Design review of the part built by this model. Coordinates are the model's own, in mm. A direction names the side the tool comes from. Coordinates: 2 decimals unless noted, no trailing zeros. Loops run counter-clockwise (first coordinate to the right, second up) from the corner with the lowest first, then second, coordinate; pieces in that order, holes last. Notation, with made-up numbers: M 40,31.25 L 76,31.25 A12 cw 76,53.25 Z; hole C 7,21 d2. An arc over 180 degrees is marked long. Put each result on its own line as item: value. Start each with the question number.
(1) Take a section at C-C, the plane z = -5.75. Give the boundary of the cut face in (x, y) (3 decimals), then the cut area to 3 significant figures.
(2) Clearance check with flat-ended pins moving along their axes: pin 1 (6 mm diameter, centred on x = -1, y = 2, fed in from +Z); pin 2 (1.5 mm diameter, centred on x = -0.5, z = 14, fed in from -Y); pin 3 (0.9 mm diameter, centred on y = 10, z = -11.5, fed in from -X); pin 4 (1.5 mm diameter, centred on y = 10.5, z = -11.5, fed in from +X). State where each tip first meets the part, or that it passes through.
(3) For probe 1 along Z at (x, y) = (-3, 7.25); probe 2 along Y at (x, z) = (1.5, -5); probe 3 along X at (y, z) = (2.2, 8), list the stretches that pass through material, from the lowest coordinate up. Write a range as [from, to].
(4) Take a section at D-D, the plane y = 10.75. Give the boundary of the cut face in (x, z).
(5) Take a section at A-A, the plane x = -5.5. Give the boundary of the cut face in (y, z), then the cut area to 3 significant figures.
(6) The part is to be moulded in two halves that separate along Z. For faces 1 (the cylindrical face through (1.142, -1.792, -0.182)), 2 (the flat face through (-2, 3.315, 7)), 3 (the flat face through (2, 2, 13)), say which applies: +Z half, -Z half, draft (parallel to the pull), parting line (faces both ways), or undercut.
(7) For faces 4 (the flat face through (-2, 11, -12)), 5 (the flat face through (0, 3.75, 14)), 6 (the cylindrical face through (-1.08, -4.88, -4.93)), list the 3-axis set-ups (+Z, -Z, +X, -X, +Y, -Y) from which the entire face can be reached by the end or side of a thin tool; tool diameter is ignored.
(8) Take a section at B-B, the plane y = -0.75. Give the boundary of the cut face in (x, z), then the cut area to 3 significant figures.
Autodesk Inventor part; units mm, degrees
ref_plane "YZ Plane" through (0, 0, 0) normal (1, 0, 0) x (0, 1, 0)
ref_plane "XZ Plane" through (0, 0, 0) normal (0, 1, 0) x (-1, 0, 0)
ref_plane "XY Plane" through (0, 0, 0) normal (0, 0, 1) x (1, 0, 0)
sketch "Sketch1" plane through (0, 0, 0) normal (0, 0, 1) x (1, 0, 0)
  circle A0 centre (0, 0) radius 5
  circle A1 centre (0, 0) radius 9
  circle A2 centre (0, 0) radius 2.125
  dimension "d0" = 10
  dimension "d1" = 18
  dimension "d2" = 4.25
extrude "Extrusion1" add sketch "Sketch1" against normal blind 10 contours A0 | A2
extrude "Extrusion2" add sketch "Sketch1" along normal blind 3 contours A0 | A1 | A2
sketch "Sketch2" plane through (0, 0, -10) normal (0, 0, -1) x (-1, 0, 0)
  circle A0 centre (0, 0) radius 9
extrude "Extrusion3" add sketch "Sketch2" along normal blind 3
sketch "Sketch3" plane through (0, 0, 3) normal (0, 0, 1) x (1, 0, 0)
  circle A0 centre (0, 0) radius 5
  circle A1 centre (0, 0) radius 2.125
  dimension "d9" = 4.25
extrude "Extrusion4" add sketch "Sketch3" along normal blind 10
ref_plane "Work Plane1" through (0, 0, -5) normal (0, 0, 1) x (1, 0, 0)
sketch "Sketch4" plane through (0, 0, -5) normal (0, 0, 1) x (1, 0, 0)
  circle A0 centre (0, 0) radius 5
  arc A1 (1.5, 4.7697) -> (-1.5, 4.7697) centre (0, 0) ccw
  line L0 (0, 0) -> (0, 5) construction
  line L1 (-1.5, 4.7697) -> (-1.5, 9.7697)
  line L2 (-1.5, 9.7697) -> (1.5, 9.7697)
  line L3 (1.5, 9.7697) -> (1.5, 4.7697)
  dimension "d12" = 5
  dimension "d13" = 3
ref_plane "Work Plane2" through (0, 5, 2) normal (0, 1, 0) x (-1, 0, 0)
sketch "Sketch5" plane through (0, 5, 2) normal (0, 1, 0) x (-1, 0, 0)
  line L0 (5, 11) -> (-5, 11)
  line L1 (-5, 1) -> (5, 1)
  line L2 (-5, 11) -> (5, 1) construction
  line L3 (5, 11) -> (-5, 1) construction
  point P0 (0, -2)
  point P1 (0, 6)
extrude "Extrusion6" cut sketch "Sketch3" against normal up to surface (16 mm away) contours A1
sketch "Sketch6" plane through (0, 5, 2) normal (0, 1, 0) x (-1, 0, 0)
  line L0 (5, 11) -> (-5, 1) construction
  line L1 (-5, 11) -> (5, 1) construction
  circle A0 centre (0, 6) radius 4
  point P0 (0, -2)
  dimension "d18" = 8
extrude "Extrusion7" add sketch "Sketch6" against normal up to surface
extrude "Extrusion8" add sketch "Sketch6" along normal blind 2.125
sketch "Sketch7" plane through (0, 7.125, 8) normal (0, 1, 0) x (1, 0, 0)
  line L0 (5, -5) -> (-5, 5) construction
  line L1 (-5, -5) -> (5, 5) construction
  circle A0 centre (0, 0) radius 4
  circle A1 centre (0, 0) radius 2.5275
  point P0 (0, 8)
  dimension "d23" = 5.055
extrude "Extrusion9" cut sketch "Sketch7" against normal blind 3.81 contours A1
sketch "Sketch8" plane through (0, 7.125, 8) normal (0, 1, 0) x (1, 0, 0)
  line L0 (-5, -5) -> (5, 5) construction
  line L1 (5, -5) -> (-5, 5) construction
  circle A0 centre (0, 0) radius 2.6545
  point P0 (0, 8)
  dimension "d26" = 5.309
loft "Loft1" cut profiles "Sketch8" section 1 edges at (-2.5275, 3.315, 8)
sketch "Sketch9" plane through (0, 3.315, 8) normal (0, 1, 0) x (1, 0, 0)
  line L0 (-5, -5) -> (5, 5) construction
  line L1 (5, -5) -> (-5, 5) construction
  circle A0 centre (0, 0) radius 1.8
  point P0 (0, 8)
  dimension "d31" = 3.6
extrude "Extrusion10" cut sketch "Sketch9" against normal up to surface
sketch "Sketch10" plane through (0, 0, -13) normal (0, 0, -1) x (-1, 0, 0)
  circle A0 centre (0, 0) radius 2.125
  circle A1 centre (0, 0) radius 9
  line L0 (0, 0) -> (0, 9) construction
  line L1 (-2, 8.775) -> (-2, 12.275)
  line L2 (-2, 12.275) -> (2, 12.275)
  line L3 (2, 12.275) -> (2, 8.775)
  arc A2 (2, 8.775) -> (-2, 8.775) centre (0, 0) ccw
  dimension "d34" = 3.5
  dimension "d35" = 4
extrude "Extrusion11" add sketch "Sketch10" against normal up to surface (3 mm away) contours A1 L1 L2 L3
sketch "Sketch12" plane through (0, 0, 13) normal (0, 0, 1) x (1, 0, 0)
  line L0 (2.1651, -3.75) -> (-2.1651, -3.75)
  line L1 (-2.1651, -3.75) -> (-4.3301, 0)
  line L2 (-4.3301, 0) -> (-2.1651, 3.75)
  line L3 (-2.1651, 3.75) -> (2.1651, 3.75)
  line L4 (2.1651, 3.75) -> (4.3301, 0)
  line L5 (4.3301, 0) -> (2.1651, -3.75)
  circle A0 centre (0, 0) radius 5
  line L6 (0, 0) -> (0, -5) construction
  circle A1 centre (0, 0) radius 5
  point P0 (0, 5)
  dimension "d39" = 7.5
extrude "Extrusion12" add sketch "Sketch12" along normal blind 3
properties part number "stationarySpindle"
Computed values:
1. outline: C 0,0 d10; hole C 0,0 d4.25
1. area: 64.4 mm^2
2. pin 1: stops at z = 16
2. pin 2: stops at y = -5
2. pin 3: stops at x = -2
2. pin 4: stops at x = 2
3. probe 1: z = [-13, -10], [0, 3]
3. probe 2: y = [-4.77, -1.51], [1.51, 4.77]
3. probe 3: x = [-4.49, -1.8], [1.8, 4.49]
4. outline: M -2,-13 L 2,-13 L 2,-10 L -2,-10 Z
5. outline: M -7.12,-13 L 7.12,-13 L 7.12,-10 L -7.12,-10 Z; M -7.12,0 L 7.12,0 L 7.12,3 L -7.12,3 Z
5. area: 85.5 mm^2
6. face 1: draft
6. face 2: undercut
6. face 3: +Z half
7. face 4: +Z, -Z, -X, +Y
7. face 5: +Z
7. face 6: none
8. outline: M -8.97,-13 L -1.99,-13 L -1.99,13 L -3.9,13 L -3.9,16 L -4.94,16 L -4.94,3 L -8.97,3 L -8.97,0 L -4.94,0 L -4.94,-10 L -8.97,-10 Z; M 1.99,-13 L 8.97,-13 L 8.97,-10 L 4.94,-10 L 4.94,0 L 8.97,0 L 8.97,3 L 4.94,3 L 4.94,16 L 3.9,16 L 3.9,13 L 1.99,13 Z
8. area: 208 mm^2
